from build123d import *

# Parameters (mm, degrees)
SKETCH011_R  = 1.45
PAD009_DEPTH = 1.5
SKETCH010_W  = 40
SKETCH010_H  = 10
SKETCH010_R  = 1.95
PAD010_DEPTH = 3
FILLET_R     = 1
FILLET001_R  = 1


with BuildPart() as part:
    # Sketch011 → Pad009 (new body, symmetric)
    with BuildSketch(Plane.XZ):
        with BuildLine():
            ThreePointArc((4, 9), (0, 13), (-4, 9))
            Line((-4, 0), (-4, 9))
            Line((4, 0), (-4, 0))
            Line((4, 9), (4, 0))
        make_face()
        with Locations((0, 9)):
            Circle(SKETCH011_R, mode=Mode.SUBTRACT)
    extrude(amount=PAD009_DEPTH, both=True)

    # Sketch010 → Pad010 (join)
    with BuildSketch(Plane.XY):
        with Locations((16, -3)):
            Rectangle(SKETCH010_W, SKETCH010_H)
        with Locations((2, -4)):
            Circle(SKETCH010_R, mode=Mode.SUBTRACT)
        with Locations((30, -4)):
            Circle(SKETCH010_R, mode=Mode.SUBTRACT)
    extrude(amount=PAD010_DEPTH)

    # Fillet
    fillet_edges = [part.edges().sort_by_distance(p)[0] for p in [
        (28.05, -4, 3),
        (0.05, -4, 3),
    ]]
    fillet(fillet_edges, radius=FILLET_R)

    # Fillet001
    fillet001_edges = [part.edges().sort_by_distance(p)[0] for p in [
        (16, -8, 3),
        (36, -3, 3),
    ]]
    fillet(fillet001_edges, radius=FILLET001_R)


solid = part.part
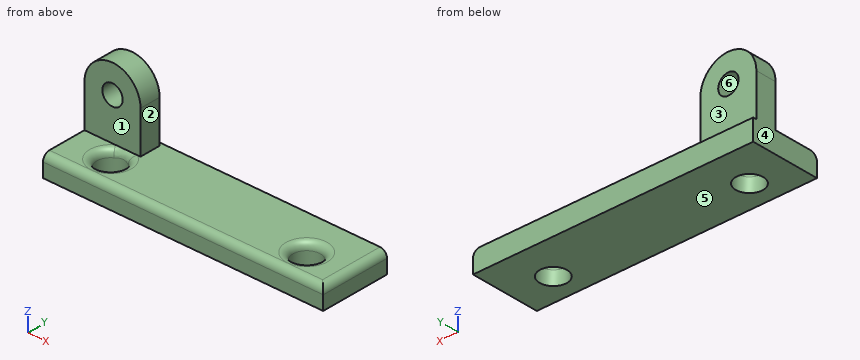
Work out the finished part from the listing and answer in its coordinate system (mm). Face numbers are marked on the shaded views. A direction names the side the tool comes from. Give positions to 0.01 mm unless a question says otherwise; leave off trailing zeros. Loops run counter-clockwise (first coordinate to the right, second up) from the corner with the lowest first, then second, coordinate; pieces in that order, holes last. Notation, with made-up numbers: (81, 40) - (110, 40) arc R24 ccw to (110, 57) - close; hole circle Ø5 at (-1.75, 38). An arc over 180 degrees is marked (long way). Answer in a Markdown table with one row per item.
(1) A tool of negligible diameter and unlimited length cuts with its end or side. For the marked faces 1, 2 and 3, from which of +Z, -Z, +X, -X, +Y, -Y can it reach the whole face along a straight path? Write none if from no direction.
Results list:
| item | result |
|---|---|
| face 1 | +Z, +X, -X, -Y |
| face 2 | +Z, +X, +Y, -Y |
| face 3 | +Z, +X, -X, +Y |
(2) Consider L1, parallel to X at y = -3.25, z = 1; L2, parallel to Y at x = 2, z = 1.4; L3, parallel to X at y = -2.25, z = 1. Determine where each line is inside the solid, lowest interval first. Write a range as [from, to].
Results list:
| item | result |
|---|---|
| L1 | x = [-4, 0.2], [3.8, 28.2], [31.8, 36] |
| L2 | y = [-8, -5.95], [-2.05, 2] |
| L3 | x = [-4, 1.14], [2.86, 29.14], [30.86, 36] |
(3) Section B-B (y = -4) is taken. Give the vertices of the cut face in (x, z), and give its area (3 significant figures).
Results list:
| item | result |
|---|---|
| outline | (-4, 0) - (0.05, 0) - (0.05, 2) arc R1 ccw to (-0.95, 3) - (-4, 3) - close; (3.95, 0) - (28.05, 0) - (28.05, 2) arc R1 ccw to (27.05, 3) - (4.95, 3) arc R1 ccw to (3.95, 2) - close; (31.95, 0) - (36, 0) - (36, 2) arc R1 ccw to (35, 3) - (32.95, 3) arc R1 ccw to (31.95, 2) - close |
| area | 95.5 mm² |
(4) Section D-D (y = 0) is taken. Give the vertices of the cut face in (x, z).
Results list:
| item | result |
|---|---|
| outline | (-4, 0) - (36, 0) - (36, 2) arc R1 ccw to (35, 3) - (4, 3) - (4, 9) arc R4 ccw to (-4, 9) - close; hole circle Ø2.9 at (0, 9) |
(5) Section C-C (x = 30) is taken. Give the vertices of the cut face in (y, z), and give its area (3 significant figures).
Results list:
| item | result |
|---|---|
| outline | (-8, 0) - (-5.95, 0) - (-5.95, 2) arc R1 ccw to (-6.95, 3) - (-7, 3) arc R1 ccw to (-8, 2) - close; (-2.05, 0) - (2, 0) - (2, 3) - (-1.05, 3) arc R1 ccw to (-2.05, 2) - close |
| area | 17.7 mm² |
(6) For a pull along X with two mould halves and no side action, classify the marked faces 4, 5 and 6 as pulls with the +X half, pulls with the -X half, needs draft (parallel to the pull), parting line crosses it, or undercut.
Results list:
| item | result |
|---|---|
| face 4 | pulls with the -X half |
| face 5 | needs draft |
| face 6 | undercut |
(7) Section A-A (z = 8) is taken. Give the vertices of the cut face in (x, y), and give its area (3 significant figures).
Results list:
| item | result |
|---|---|
| outline | (-4, -1.5) - (-1.05, -1.5) - (-1.05, 1.5) - (-4, 1.5) - close; (1.05, -1.5) - (4, -1.5) - (4, 1.5) - (1.05, 1.5) - close |
| area | 17.7 mm² |
(8) Flat-ended cylindrical pins translate along their axes: pin 1 Ø6.5 at (x, z) = (-0.5, 8.5) entering from -Y; pin 2 Ø1.5 at (x, z) = (28, 3.5) entering from -Y; pin 3 Ø4.5 at (x, z) = (0, 9) entering from +Y. Find the tip coordinate at first contact, or state that the pin passes through.
Results list:
| item | result |
|---|---|
| pin 1 | stops at y = -1.5 |
| pin 2 | stops at y = -7.66 |
| pin 3 | stops at y = 1.5 |
